Answer from the drawing. Dimensions are ordinates in mm from the lowest x, y and z of the part. Give positions to 0.01 mm unless a question says otherwise; leave off trailing zeros. Loops run counter-clockwise (first coordinate to the right, second up) from the corner with the lowest first, then second, coordinate; pieces in that order, holes last.
(1) Find section D-D, the plane x = 45.5. Write down the section's boundary in (y, z), then the cut area to 3 significant figures.
(2) Each of these flat-tipped pins is pushed along its axis until it touches: P1, Ø2, axis at x = 22.5, y = 1, coming from the +Z side; P2, Ø1, axis at x = 44.5, y = 2, coming from the -Z side; P3, Ø1, axis at x = 19.5, y = 1, coming from the -Z side. Where does it stop, or does it pass through?
(3) Straight lines are drawn through the part: probe 1 along Z at (x, y) = (5, 2.9); probe 2 along X at (y, z) = (1.4, 28); probe 3 along X at (y, z) = (1.85, 51.44). For each, find the intervals that lie inside material, in ascending order.
(4) Determine the mould class of the marked faces 1, 2, 3 and 4 for opening direction Z: pulls with the +Z half, pulls with the -Z half, needs draft (parallel to the pull), parting line crosses it, or undercut.
(5) Find section C-C, the plane y = 2.7. Write down the section's boundary in (x, z), then the cut area to 3 significant figures.
(6) Find section B-B, the plane x = 51.44. Write down the section's boundary in (y, z).
(7) Find section A-A, the plane z = 51.44. Write down the section's boundary in (x, y), then the cut area to 3 significant figures.
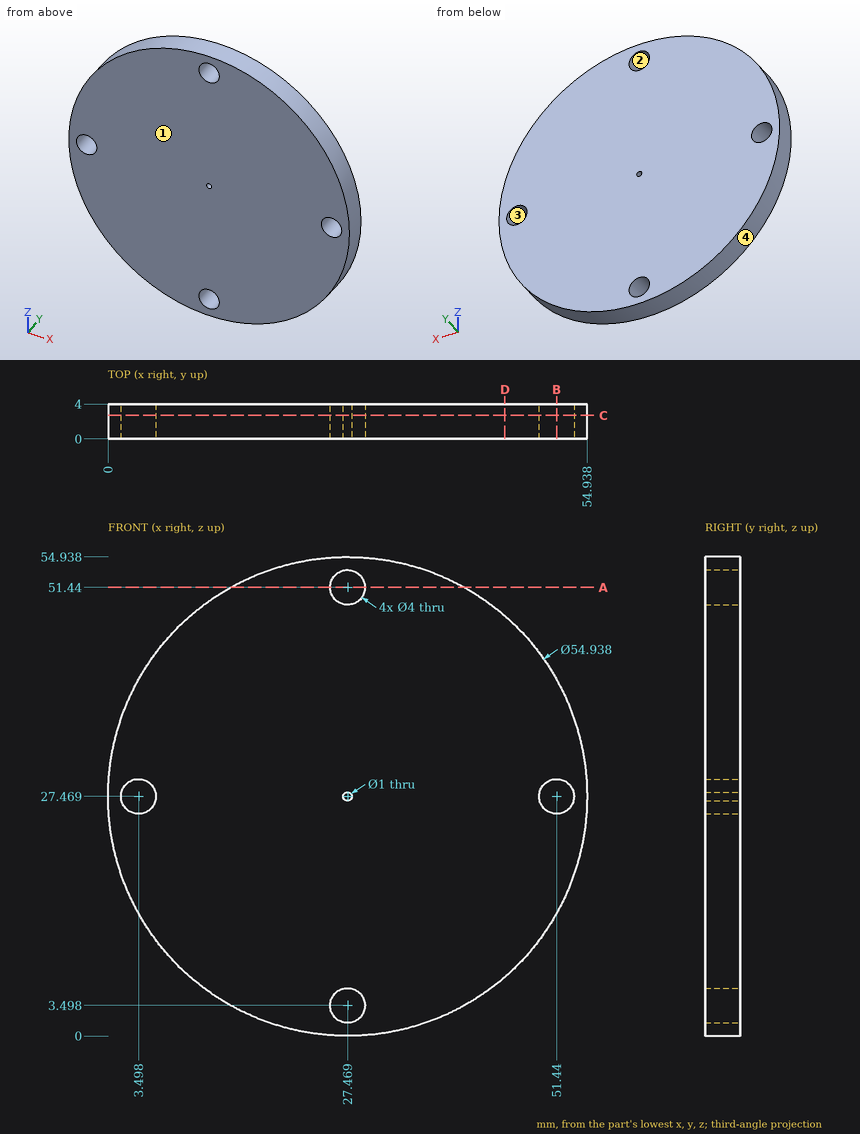
Entries:
1. outline: (0, 6.75) - (4, 6.75) - (4, 48.19) - (0, 48.19) - close
1. area: 166 mm2
2. P1: stops at z = 54.65
2. P2: stops at z = 5.53
2. P3: stops at z = 1.03
3. probe 1: z = 11.67 to 26.15, 28.79 to 43.27
3. probe 2: x = 0.01 to 1.57, 5.43 to 49.51, 53.37 to 54.93
3. probe 3: x = 14.05 to 25.47, 29.47 to 40.88
4. face 1: needs draft
4. face 2: undercut
4. face 3: undercut
4. face 4: parting line crosses it
5. outline: circle Ø54.94 at (27.47, 27.47); hole circle Ø4 at (3.5, 27.47); hole circle Ø4 at (27.47, 3.5); hole circle Ø4 at (27.47, 51.44); hole circle Ø1 at (27.47, 27.47); hole circle Ø4 at (51.44, 27.47)
5. area: 2,320 mm2
6. outline: (0, 14.05) - (4, 14.05) - (4, 25.47) - (0, 25.47) - close; (0, 29.47) - (4, 29.47) - (4, 40.88) - (0, 40.88) - close
7. outline: (14.05, 0) - (25.47, 0) - (25.47, 4) - (14.05, 4) - close; (29.47, 0) - (40.88, 0) - (40.88, 4) - (29.47, 4) - close
7. area: 91.3 mm2
